Autodesk Inventor part; units mm, degrees
ref_plane "Work Plane2" through (2.032, 0, 0) normal (0, 1, 0) x (1, 0, 0)
ref_plane "YZ Plane" through (0, 0, 0) normal (1, 0, 0) x (0, 1, 0)
ref_plane "XZ Plane" through (0, 0, 0) normal (0, 1, 0) x (-1, 0, 0)
sketch "Sketch1" plane through (0, 0, 0) normal (0, 0, 1) x (1, 0, 0)
  line L0 (6.6294, 0) -> (15.875, 0)
  line L1 (15.875, 0) -> (15.875, 5.5563)
  line L2 (15.875, 5.5563) -> (5.6642, 5.5563)
  line L3 (1.4931, 9.1821) -> (0, 9.1821)
  line L4 (-3.175, 0) -> (19.05, 0)
  line L5 (0, -1.8364) -> (0, 11.0185)
  line L6 (0, 5.1943) -> (5.2627, 2.5704)
  line L7 (5.2627, 2.5704) -> (6.6294, 0)
  line L8 (5.6642, 5.5563) -> (1.4931, 9.1821)
  line L9 (0, 9.1821) -> (0, 5.1943)
  dimension "d2" = 11.1125
  dimension "d3" = 18.3642
  dimension "d4" = 6.6294
  dimension "d5" = 10.3886
  dimension "d6" = 26.5
  dimension "d7" = 62
  dimension "d13" = 41
  dimension "d14" = 5.6642
  dimension "d15" = 15.875
revolve "Body" add sketch "Sketch1" angle 360 about axis through (6.6294, 0, 0) along (1, 0, 0) contours L7 L6 L5 L3 L8 L2 L1 L0
sketch "Sketch2" plane through (0, 0, 0) normal (-1, 0, 0) x (0, 0, 1)
  line L0 (0, -12.8549) -> (0, 12.8549)
  line L1 (-12.8549, 0) -> (12.8549, 0)
  line L2 (0, 5.1943) -> (0, 0) construction
  line L3 (0, 0) -> (5.1943, 0) construction
  arc A0 (1.7314, 0) -> (0, 1.7314) centre (0, 0) ccw
  line L4 (0, 0) -> (0.7947, 0.7947) construction
  arc A1 (2.5971, 0) -> (0, 2.5971) centre (0, 0) ccw construction
  line L5 (0.8636, 5.122) -> (0.7354, 2.4908)
  line L6 (5.122, 0.8636) -> (2.4908, 0.7354)
  arc A2 (0.7354, 2.4908) -> (2.4908, 0.7354) centre (2.4093, 2.4093) ccw
  arc A3 (5.1943, 0) -> (5.122, 0.8636) centre (0, 0) ccw
  arc A4 (0.8636, 5.122) -> (0, 5.1943) centre (0, 0) ccw
  arc A5 (5.122, 0.8636) -> (0.8636, 5.122) centre (0, 0) ccw
  line L7 (0.8636, -5.122) -> (0.7354, -2.4908)
  line L8 (5.122, -0.8636) -> (2.4908, -0.7354)
  arc A6 (2.4908, -0.7354) -> (0.7354, -2.4908) centre (2.4093, -2.4093) ccw
  arc A7 (5.122, -0.8636) -> (5.1943, 0) centre (0, 0) ccw
  arc A8 (0, -5.1943) -> (0.8636, -5.122) centre (0, 0) ccw
  arc A9 (0.8636, -5.122) -> (5.122, -0.8636) centre (0, 0) ccw
  line L9 (-0.8636, 5.122) -> (-0.7354, 2.4908)
  line L10 (-5.122, 0.8636) -> (-2.4908, 0.7354)
  arc A10 (-2.4908, 0.7354) -> (-0.7354, 2.4908) centre (-2.4093, 2.4093) ccw
  arc A11 (-5.122, 0.8636) -> (-5.1943, 0) centre (0, 0) ccw
  arc A12 (0, 5.1943) -> (-0.8636, 5.122) centre (0, 0) ccw
  arc A13 (-0.8636, 5.122) -> (-5.122, 0.8636) centre (0, 0) ccw
  arc A14 (-5.122, -0.8636) -> (-0.8636, -5.122) centre (0, 0) ccw
  arc A15 (-0.8636, -5.122) -> (0, -5.1943) centre (0, 0) ccw
  arc A16 (-5.1943, 0) -> (-5.122, -0.8636) centre (0, 0) ccw
  line L11 (-5.122, -0.8636) -> (-2.4908, -0.7354)
  arc A17 (-0.7354, -2.4908) -> (-2.4908, -0.7354) centre (-2.4093, -2.4093) ccw
  line L12 (-0.8636, -5.122) -> (-0.7354, -2.4908)
  dimension "d18" = 45
  dimension "d19" = 3.4629
  dimension "d20" = 5.1943
  dimension "d21" = 10.3886
  dimension "d22" = 0.8636
extrude "Slot" add sketch "Sketch2" against normal up to next contours A2 L5 A5 L6 | L9 A10 L10 A13 | L7 A6 L8 A9 | A14 L11 A17 L12
fillet "Fillet1" radius 0.3454 4 edges at (0, 5.1943, 0) (0, 0, 5.1943) (0, -5.1943, 0) (0, 0, -5.1943)
thread "Thread"
chamfer "Chamfer1" distance 1.3606 distance2 1.3606 1 edges at (15.875, -5.5563, 0) measured on face at (15.875, 2.9153, 1.1751)
ref_plane "Work Plane2" through (2.032, 0, 0) normal (0, 1, 0) x (1, 0, 0)
equation "\"d2\" = GD"
equation "\"d3\" = KOD"
equation "\"d4\" = INTI"
equation "\"d5\" = SDM"
equation "\"d13\" = 0.5 * SEWI"
equation "\"d14\" = KOH"
equation "\"d15\" = NLG"
equation "\"d19\" = 0.333333 * SDM"
equation "\"d20\" = 0.5 * SDM"
equation "\"d21\" = SDM"
equation "\"d22\" = 0.5 * SBR"
equation "\"d45\" = INTI"
equation "\"d25\" = 0.2 * SBR"
equation "\"d9\" = GEL"
equation "\"d11\" = -0.5 * SPD + 0.5 * GD"
equation "\"d12\" = GUL"
equation "\"GD\" = NND"
equation "\"NLG\" = 15.875"
equation "\"GEL\" = 5.67563"
equation "\"KOD\" = 18.3642"
equation "\"KOH\" = 5.6642"
equation "\"SDM\" = 10.3886"
equation "\"INTI\" = 6.6294"
equation "\"SBR\" = 1.7272"
equation "\"GUL\" = 0.75 * GAL"
equation "\"SPD\" = 8.3914"
equation "\"SEWI\" = 82deg"
equation "\"d0\" = NLG"
equation "\"d1\" = KOH"
equation "\"d17\" = SDM"
equation "\"TOA\" = 30deg"
equation "\"THREADDIA\" = 11.1125"
equation "\"BDM\" = NND"
equation "\"NND\" = 11.1125"
equation "\"GAL\" = 1.81407"
equation "\"GD1\" = SPD"
properties part number "ANSI B18.6.3 - 7/16-14 x 5/8, CRFCHMSTII(5)" material "Steel, Mild"
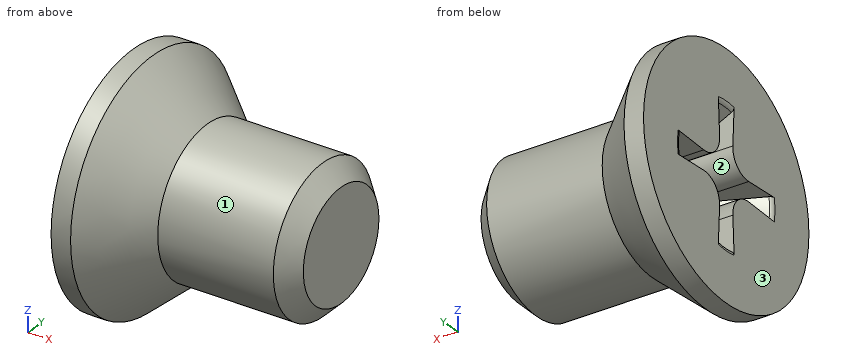
Verification items for the finished model (mm, model axes). Face numbers are marked on the shaded views. A direction names the side the tool comes from. Give positions to 0.01 mm unless a question says otherwise; leave off trailing zeros. Order: outer loops, then holes, each group sorted by start corner. A loop starts at its lowest first (then second) coordinate and runs counter-clockwise, first axis right, second up. Notation, with made-up numbers: M 25,1 L 65,1 A32 ccw 65,33 Z; hole C 63,6.5 d11. An arc over 180 degrees is marked long. Answer in a Markdown table with one row per item. Add a question column.
Item 1: Tool access check on the marked faces 1, 2 and 3. Record the directions out of +Z, -Z, +X, -X, +Y, -Y that give a thin tool (end or side, any length) a straight path to the whole face; none if there is none.
Item 2: Gauge pin test, flat ends, axial feed: pin 1 (2 mm diameter, centred on x = 3.5, y = -7, fed in from -Z); pin 2 (1 mm diameter, centred on x = 5.5, z = 2.5, fed in from -Y); pin 3 (3 mm diameter, centred on x = 12.5, z = 6, fed in from +Y). Record the tip position at first contact, or that the pin passes through.
Item 3: Section check A-A, the plane x = 2. Enter the section's corners in (y, z), and give its area (3 significant figures).
Item 4: Section check B-B, the plane x = 9.25. Enter the section's corners in (y, z).
Item 5: Scan lines: probe 1 along Z at (x, y) = (3.5, -3); probe 2 along Y at (x, z) = (3, 1.75); probe 3 along X at (y, z) = (6, 1.5). Record each from-to range of solid material in increasing order. Write a range as from..to.
Item 6: Section check C-C, the plane x = 4.5. Enter the section's corners in (y, z).
Filled sheet:
| question | item | result |
|---|---|---|
| 1 | face 1 | +X |
| 1 | face 2 | -X |
| 1 | face 3 | +Z, -Z, -X, +Y, -Y |
| 2 | pin 1 | stops at z = -5.03 |
| 2 | pin 2 | stops at y = -5.65 |
| 2 | pin 3 | stops at y = 3.26 |
| 3 | outline | C 0,0 d17.48; hole M -4.12,-0.81 L -2.49,-0.74 A1.68 cw -0.74,-2.49 L -0.81,-4.12 A4.2 ccw 0.81,-4.12 L 0.74,-2.49 A1.68 cw 2.49,-0.74 L 4.12,-0.81 A4.2 ccw 4.12,0.81 L 2.49,0.74 A1.68 cw 0.74,2.49 L 0.81,4.12 A4.2 ccw -0.81,4.12 L -0.74,2.49 A1.68 cw -2.49,0.74 L -4.12,0.81 A4.2 ccw Z |
| 3 | area | 215 mm^2 |
| 4 | outline | C 0,0 d11.11 |
| 5 | probe 1 | z = -6.81..-0.76, 0.76..6.81 |
| 5 | probe 2 | y = -7.68..-0.87, 0.87..7.68 |
| 5 | probe 3 | x = 0..4.94 |
| 6 | outline | C 0,0 d13.14; hole M -2.85,-0.75 L -2.49,-0.74 A1.68 cw -0.74,-2.49 L -0.75,-2.85 A2.95 ccw 0.75,-2.85 L 0.74,-2.49 A1.68 cw 2.49,-0.74 L 2.85,-0.75 A2.95 ccw 2.85,0.75 L 2.49,0.74 A1.68 cw 0.74,2.49 L 0.75,2.85 A2.95 ccw -0.75,2.85 L -0.74,2.49 A1.68 cw -2.49,0.74 L -2.85,0.75 A2.95 ccw Z |
